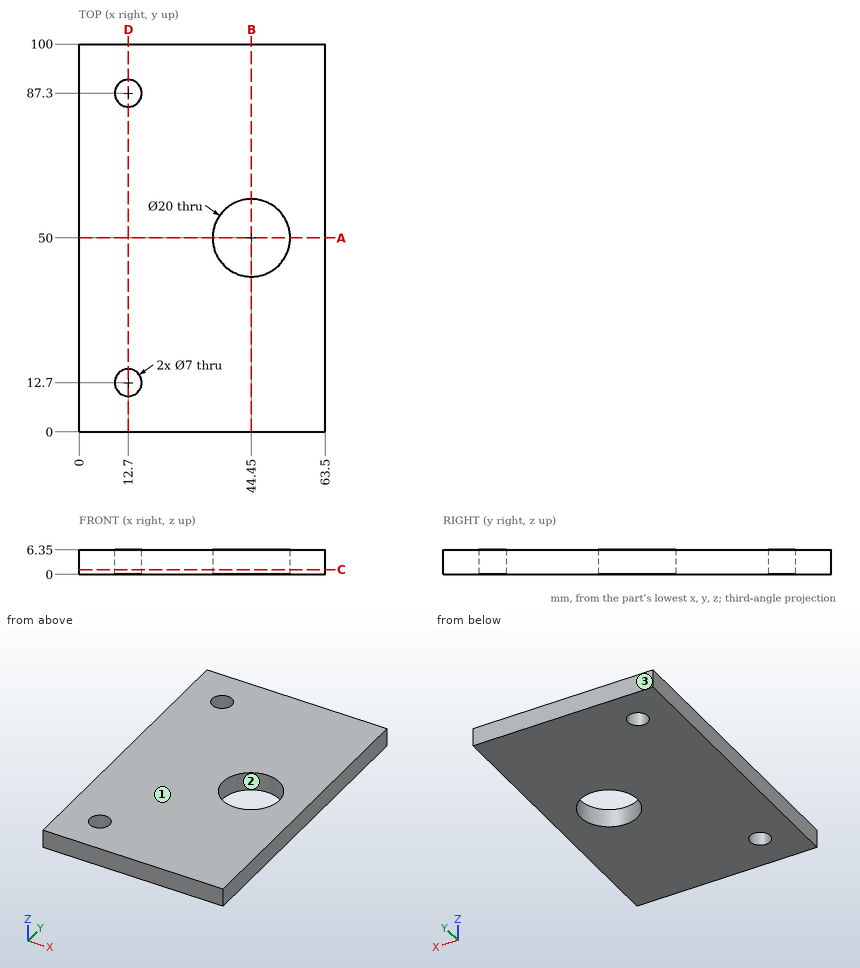
Source: three-view drawing plus pictorial views. Frame: mm from the lowest corner of the part. Round coordinates to 2 decimals unless told otherwise and drop trailing zeros. Write each loop counter-clockwise with the first axis right and the second up, starting at its lowest first coordinate (ties: lowest second). Pieces come first, ordered by that corner, then holes. Notation, with made-up numbers: M 7,0.5 L 58,0.5 A19 ccw 58,8.5 Z; hole C -31,67 d4. An arc over 180 degrees is marked long. Write item = value, one per line.
Item 1: Pin query (flat end, axial travel): P1, Ø5.5, axis at x = 12.7, y = 12.7, coming from the -Z side. Return the tip coordinate at first contact, or that it passes through.
Findings:
P1 = through
Item 2: Section query C-C on z = 1.25. Return loops of the section in (x, y).
Findings:
outline = M 0,0 L 63.5,0 L 63.5,100 L 0,100 Z; hole C 12.7,12.7 d7; hole C 12.7,87.3 d7; hole C 44.45,50 d20
Item 3: Section query B-B on x = 44.45. Return loops of the section in (y, z), then the cut area to 3 significant figures.
Findings:
outline = M 0,0 L 40,0 L 40,6.35 L 0,6.35 Z; M 60,0 L 100,0 L 100,6.35 L 60,6.35 Z
area = 508 mm^2
Item 4: Section query D-D on x = 12.7. Return loops of the section in (y, z), then the cut area to 3 significant figures.
Findings:
outline = M 0,0 L 9.2,0 L 9.2,6.35 L 0,6.35 Z; M 16.2,0 L 83.8,0 L 83.8,6.35 L 16.2,6.35 Z; M 90.8,0 L 100,0 L 100,6.35 L 90.8,6.35 Z
area = 546 mm^2
Item 5: Material intervals for line 1 along Y through (x, z) = (12.7, 5.25); line 2 along Y through (x, z) = (44.45, 4.5); line 3 along X through (y, z) = (87.3, 4.25), sorted ascending. Write a range as [from, to].
Findings:
line_1 = [0, 9.2], [16.2, 83.8], [90.8, 100]
line_2 = [0, 40], [60, 100]
line_3 = [0, 9.2], [16.2, 63.5]
Item 6: Section query A-A on y = 50. Return loops of the section in (x, z).
Findings:
outline = M 0,0 L 34.45,0 L 34.45,6.35 L 0,6.35 Z; M 54.45,0 L 63.5,0 L 63.5,6.35 L 54.45,6.35 Z
Item 7: Pull-direction query (Y, two-part tool) for the marked faces 1, 2 and 3; classes: pulls with the +Y half, pulls with the -Y half, needs draft (parallel to the pull), parting line crosses it, or undercut.
Findings:
face_1 = needs draft
face_2 = undercut
face_3 = pulls with the +Y half
